Work out the finished part from the listing and answer in its coordinate system (mm). A direction names the side the tool comes from. Coordinates: 2 decimals unless noted, no trailing zeros. Write each loop counter-clockwise with the first axis right and the second up, starting at its lowest first coordinate (ties: lowest second). Pieces come first, ordered by that corner, then holes. Notation, with made-up numbers: (27.25, 32) - (49.25, 32) arc R26 cw to (49.25, 56) - close; hole circle Ø6 at (-26.5, -17.5). An arc over 180 degrees is marked (long way). One line per item, written item: value.
```python
from build123d import *


with BuildPart() as part:
    # Croquis1 → Revolución1 (revolve)
    with BuildSketch(Plane.XY):
        with BuildLine():
            Line((3.5, 46.282828283), (6, 46.282828283))
            Line((6, 46.282828283), (6, 36.282828283))
            Line((6, 36.282828283), (7, 36.282828283))
            Line((7, 36.282828283), (7, 35.032828283))
            Line((7, 35.032828283), (9.5, 35.032828283))
            Line((9.5, 35.032828283), (9.5, 36.282828283))
            Line((9.5, 36.282828283), (11, 36.282828283))
            Line((11, 36.282828283), (11, -82.217171717))
            Line((11, -82.217171717), (7, -82.217171717))
            Line((7, -82.217171717), (7, -114.217171717))
            Line((7, -114.217171717), (5.161616162, -114.217171717))
            Line((5.161616162, -114.217171717), (5.161616162, -117.217171717))
            Line((5.161616162, -117.217171717), (6.080808081, -116.297979798))
            Line((6.080808081, -116.297979798), (6.080808081, -144.297979798))
            ThreePointArc((6.080808081, -144.297979798), (5.811583001, -144.947946637), (5.161616162, -145.217171717))
            Line((5.161616162, -145.217171717), (0, -145.217171717))
            Line((0, -145.217171717), (0, 21.282828283))
            Line((0, 21.282828283), (3.5, 21.282828283))
            Line((3.5, 21.282828283), (3.5, 46.282828283))
        make_face()
    revolve(axis=Axis((0, 29.484848485, 0), (0, -1, 0)))


solid = part.part
```
Item 1: Given pin 1 (2 mm diameter, centred on x = -2, z = 0, fed in from +Y); pin 2 (6.5 mm diameter, centred on x = -1.5, z = 1.5, fed in from +Y); pin 3 (12 mm diameter, centred on y = -122, z = -8, fed in from -X); pin 4 (6 mm diameter, centred on y = -27, z = 4, fed in from -X), each flat-ended and moving along its own axis, determine where each tip first touches the part or whether it passes through.
Evaluation:
pin 1: stops at y = 21.28
pin 2: stops at y = 46.28
pin 3: stops at x = -5.74
pin 4: stops at x = -10.95
Item 2: Determine the mould class of faces 1 (the face through (0, 21.283, 0)), 2 (the face through (-6, 36.283, 2)), 3 (the face through (-2.38, -23.8, -10.74)) for opening direction X: +X half, -X half, draft (parallel to the pull), parting line (faces both ways), or undercut.
Evaluation:
face 1: undercut
face 2: draft
face 3: parting line
Item 3: Section D-D, the plane y = -89.5 is taken. Determine the outline of the cut face in (x, z).
Evaluation:
outline: circle Ø14 at (0, 0)
Item 4: Which of the six approach directions +Z, -Z, +X, -X, +Y, -Y give full straight-line access (tool end or side, diameter ignored) to faces 4 (the face through (10, 36.283, 0)), 5 (the face through (-3, -114.217, -5)), 6 (the face through (-6.075, -130.494, 0.267))?
Evaluation:
face 4: +Y
face 5: none
face 6: -Y
Item 5: Consider probe 1 along Z at (x, y) = (0, 35.7); probe 2 along Z at (x, y) = (0, 35); probe 3 along Y at (x, z) = (-3, 6.5). Determine where each line is inside the solid, lowest interval first.
Evaluation:
probe 1: z = -11 to -9.5, -7 to -3.5, 3.5 to 7, 9.5 to 11
probe 2: z = -11 to -3.5, 3.5 to 11
probe 3: y = -82.22 to 35.03
Item 6: Section C-C, the plane y = 30 is taken. Determine the outline of the cut face in (x, z), then the cut area to 3 significant figures.
Evaluation:
outline: circle Ø22 at (0, 0); hole circle Ø7 at (0, 0)
area: 342 mm2
